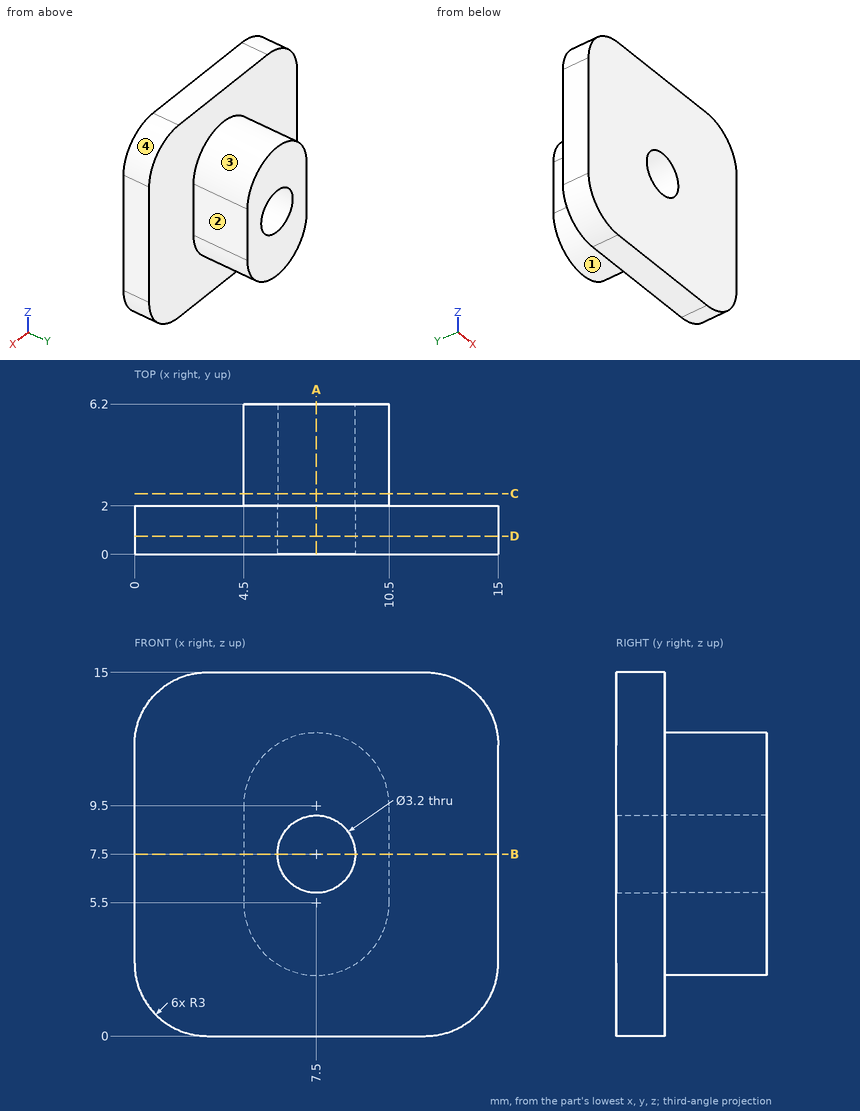
Geometry check sheet. Reference: drawing and pictorial views, mm from the part's lowest x, y, z. A direction names the side the tool comes from. Coordinates: 2 decimals unless noted, no trailing zeros. Order: outer loops, then holes, each group sorted by start corner. A loop starts at its lowest first (then second) coordinate and runs counter-clockwise, first axis right, second up. Notation, with made-up numbers: (32, -23.75) - (68, -23.75) arc R20 cw to (68, -3.75) - close; hole circle Ø10 at (-10, -15.75). An arc over 180 degrees is marked (long way). Answer in a Markdown table with one row per item. Add a question column.
1) Cross-section at C-C, the plane y = 2.5. Record the cut outline in (x, z).
2) Gauge pin test, flat ends, axial feed: P1, Ø1.5, axis at x = 9.5, z = 3.5, coming from the -Y side; P2, Ø2, axis at y = 5, z = 5, coming from the +X side. Record the tip position at first contact, or that the pin passes through.
3) Set-up check for the marked faces 1, 2, 3 and 4: record each of +Z, -Z, +X, -X, +Y, -Y from which the full face is reachable in a straight line by a thin tool's end or side.
4) Cross-section at A-A, the plane x = 7.5. Record the cut outline in (y, z), then the cut area to 3 significant figures.
5) Material ranges on line 1 along X through (y, z) = (3.15, 7.5); line 2 along X through (y, z) = (0.6, 7.5); line 3 along Z through (x, y) = (7.5, 3.6), recorded low to high. Write a range as [from, to].
6) Cross-section at B-B, the plane z = 7.5. Record the cut outline in (x, y), then the cut area to 3 significant figures.
7) Cross-section at D-D, the plane y = 0.75. Record the cut outline in (x, z), then the cut area to 3 significant figures.
Check result:
| question | item | result |
|---|---|---|
| 1 | outline | (4.5, 5.5) arc R3 ccw to (10.5, 5.5) - (10.5, 9.5) arc R3 ccw to (4.5, 9.5) - close; hole circle Ø3.2 at (7.5, 7.5) |
| 2 | P1 | stops at y = 0 |
| 2 | P2 | stops at x = 10.5 |
| 3 | face 1 | -Z, +Y |
| 3 | face 2 | +Z, -Z, +X, +Y |
| 3 | face 3 | +Z, +Y |
| 3 | face 4 | +Z, +X, +Y, -Y |
| 4 | outline | (0, 0) - (2, 0) - (2, 2.5) - (6.2, 2.5) - (6.2, 5.9) - (0, 5.9) - close; (0, 9.1) - (6.2, 9.1) - (6.2, 12.5) - (2, 12.5) - (2, 15) - (0, 15) - close |
| 4 | area | 52.2 mm² |
| 5 | line 1 | x = [4.5, 5.9], [9.1, 10.5] |
| 5 | line 2 | x = [0, 5.9], [9.1, 15] |
| 5 | line 3 | z = [2.5, 5.9], [9.1, 12.5] |
| 6 | outline | (0, 0) - (5.9, 0) - (5.9, 6.2) - (4.5, 6.2) - (4.5, 2) - (0, 2) - close; (9.1, 0) - (15, 0) - (15, 2) - (10.5, 2) - (10.5, 6.2) - (9.1, 6.2) - close |
| 6 | area | 35.4 mm² |
| 7 | outline | (0, 3) arc R3 ccw to (3, 0) - (12, 0) arc R3 ccw to (15, 3) - (15, 12) arc R3 ccw to (12, 15) - (3, 15) arc R3 ccw to (0, 12) - close; hole circle Ø3.2 at (7.5, 7.5) |
| 7 | area | 209 mm² |
